from build123d import *

# Parameters (mm, degrees)
SKETCH1_W                    = 20
SKETCH1_H                    = 15
SKETCH1_W_2                  = 40
SKETCH1_H_2                  = 10
BOSS_EXTRUDE1_DEPTH          = 5
M3_CLEARANCE_HOLE1_OUTLINE_R = 1.7
M3_CLEARANCE_HOLE1_DEPTH     = 5
SKETCH4_W                    = 17
SKETCH4_H                    = 10
BOSS_EXTRUDE2_DEPTH          = 5
HOLE1_OUTLINE_R              = 2.2
HOLE1_DEPTH                  = 3
HOLE1_START                  = 3
HOLE1_2_OUTLINE_R            = 1.7
HOLE1_2_DEPTH                = 2
FILLET1_R                    = 4
FILLET2_R                    = 0.8


# Read off the part's stored shape, not the designer's step: M3 Clearance Hole1, Hole1
with BuildPart() as part:
    # Sketch1 → Boss-Extrude1 (new body)
    with BuildSketch(Plane.XY):
        with Locations((10, 17.5)):
            Rectangle(SKETCH1_W, SKETCH1_H)
        with Locations((20, 5)):
            Rectangle(SKETCH1_W_2, SKETCH1_H_2)
    extrude(amount=BOSS_EXTRUDE1_DEPTH)

    # M3 Clearance Hole1 outline → M3 Clearance Hole1 (cut)
    with BuildSketch(Plane.XY):
        with Locations((5, 17.5)):
            Circle(M3_CLEARANCE_HOLE1_OUTLINE_R)
        with Locations((15, 17.5)):
            Circle(M3_CLEARANCE_HOLE1_OUTLINE_R)
        with Locations((15, 5)):
            Circle(M3_CLEARANCE_HOLE1_OUTLINE_R)
        with Locations((35, 5)):
            Circle(M3_CLEARANCE_HOLE1_OUTLINE_R)
    extrude(amount=M3_CLEARANCE_HOLE1_DEPTH, mode=Mode.SUBTRACT)

    # Sketch4 → Boss-Extrude2 (add)
    with BuildSketch(Plane.XY.offset(5)):
        with Locations((-8.5, 5)):
            Rectangle(SKETCH4_W, SKETCH4_H)
    extrude(amount=-BOSS_EXTRUDE2_DEPTH)

    # Hole1 outline → Hole1 (cut)
    with BuildSketch(Plane.XY):
        with Locations((8, 5)):
            Circle(HOLE1_OUTLINE_R)
        with Locations((-12, 5)):
            Circle(HOLE1_OUTLINE_R)
    extrude(amount=HOLE1_DEPTH, mode=Mode.SUBTRACT)

    # Hole1 2 outline → Hole1 2 (cut)
    with BuildSketch(Plane.XY.offset(HOLE1_START)):
        with Locations((8, 5)):
            Circle(HOLE1_2_OUTLINE_R)
        with Locations((-12, 5)):
            Circle(HOLE1_2_OUTLINE_R)
    extrude(amount=HOLE1_2_DEPTH, mode=Mode.SUBTRACT)

    # Fillet1
    fillet1_edges = [part.edges().sort_by_distance(p)[0] for p in [
        (0, 25, 2.5),
        (20, 25, 2.5),
        (20, 10, 2.5),
        (40, 10, 2.5),
        (40, 0, 2.5),
        (0, 10, 2.5),
        (-17, 0, 2.5),
        (-17, 10, 2.5),
    ]]
    fillet(fillet1_edges, radius=FILLET1_R)

    # Fillet2
    fillet2_edges = [part.edges().sort_by_distance(p)[0] for p in [
        (21.171572875, 11.171572875, 0),
        (21.171572875, 11.171572875, 5),
        (-1.171572875, 11.171572875, 5),
        (-1.171572875, 11.171572875, 0),
        (-17, 5, 0),
        (-17, 5, 5),
        (0, 17.5, 5),
        (-8.5, 10, 5),
        (11.5, 0, 5),
        (40, 5, 5),
        (30, 10, 5),
        (20, 17.5, 5),
        (10, 25, 5),
        (1.171572875, 23.828427125, 5),
        (18.828427125, 23.828427125, 5),
        (38.828427125, 8.828427125, 5),
        (38.828427125, 1.171572875, 5),
        (-15.828427125, 8.828427125, 5),
        (-15.828427125, 1.171572875, 5),
        (11.5, 0, 0),
        (-8.5, 10, 0),
        (0, 17.5, 0),
        (10, 25, 0),
        (20, 17.5, 0),
        (30, 10, 0),
        (40, 5, 0),
        (1.171572875, 23.828427125, 0),
        (18.828427125, 23.828427125, 0),
        (38.828427125, 8.828427125, 0),
        (38.828427125, 1.171572875, 0),
        (-15.828427125, 8.828427125, 0),
        (-15.828427125, 1.171572875, 0),
    ]]
    fillet(fillet2_edges, radius=FILLET2_R)


solid = part.part
Part model, mm, in its own coordinate system. A direction names the side the tool comes from. Give positions to 0.01 mm unless a question says otherwise; leave off trailing zeros. Loops run counter-clockwise (first coordinate to the right, second up) from the corner with the lowest first, then second, coordinate; pieces in that order, holes last. Notation, with made-up numbers: M -23.5,30 L 18.5,30 A26 cw 18.5,59 Z; hole C 87.5,-4 d5. An arc over 180 degrees is marked long. Put each result on its own line as item: value. Start each with the question number.
1) Probe probe 1 along Y at (x, z) = (14.5, 4.65); probe 2 along Y at (x, z) = (15, 3.35); probe 3 along X at (y, z) = (4.25, 1.35). List the from-to ranges inside material, lowest first.
2) Pull direction X, two halves, no side cores. Call faces 1 (the flat face through (6, 5, 3)), 2 (the flat face through (11, 0, 3)), 3 (the flat face through (-17, 5, 3)): +X half, -X half, draft (parallel to the pull), parting line (faces both ways), or undercut.
3) Saw through at A-A (x = 5). List the corners of the cut face in (y, z).
4) Saw through at C-C (x = 15). List the corners of the cut face in (y, z).
5) Saw through at D-D (y = 17.5). List the corners of the cut face in (x, z), then the cut area to 3 significant figures.
6) 3-axis set-ups, long thin cutter, end or side, ignore diameter. For faces 4 (the cylindrical face through (-9.968, 4.157, 1.479)), 5 (the flat face through (11, 10, 0)): which of +Z, -Z, +X, -X, +Y, -Y reach the whole face in a straight line?
7) Flat gauge pins, fed straight in: pin 1 (2.5 mm diameter, centred on x = 8, y = 5, fed in from +Z); pin 2 (1 mm diameter, centred on y = 16.5, z = 3, fed in from -X); pin 3 (4 mm diameter, centred on x = 15, y = 5, fed in from +Z); pin 4 (2.5 mm diameter, centred on x = 28.5, z = 2, fed in from +Y). Where does each tip first touch, or does it go through?
8) Saw through at B-B (y = 5). State how many separate pieces and enclosed holes the cut face has, then the cut area to 3 significant figures.
Numbers:
1. probe 1: 0.14 to 3.38, 6.62 to 15.88, 19.12 to 24.86
1. probe 2: 0 to 3.3, 6.7 to 15.8, 19.2 to 25
1. probe 3: -17 to -14.07, -9.93 to 5.93, 10.07 to 13.47, 16.53 to 33.47, 36.53 to 40
2. face 1: undercut
2. face 2: draft
2. face 3: -X half
3. outline: M 0,0.8 A0.8 ccw 0.8,0 L 15.8,0 L 15.8,5 L 0.8,5 A0.8 ccw 0,4.2 Z; M 19.2,0 L 24.2,0 A0.8 ccw 25,0.8 L 25,4.2 A0.8 ccw 24.2,5 L 19.2,5 Z
4. outline: M 0,0.8 A0.8 ccw 0.8,0 L 3.3,0 L 3.3,5 L 0.8,5 A0.8 ccw 0,4.2 Z; M 6.7,0 L 15.8,0 L 15.8,5 L 6.7,5 Z; M 19.2,0 L 24.2,0 A0.8 ccw 25,0.8 L 25,4.2 A0.8 ccw 24.2,5 L 19.2,5 Z
5. outline: M 0,0.8 A0.8 ccw 0.8,0 L 3.3,0 L 3.3,5 L 0.8,5 A0.8 ccw 0,4.2 Z; M 6.7,0 L 13.3,0 L 13.3,5 L 6.7,5 Z; M 16.7,0 L 19.2,0 A0.8 ccw 20,0.8 L 20,4.2 A0.8 ccw 19.2,5 L 16.7,5 Z
5. area: 65.5 mm^2
6. face 4: -Z
6. face 5: -Z, +X, -X, +Y, -Y
7. pin 1: through
7. pin 2: x = 0
7. pin 3: z = 5
7. pin 4: y = 10
8. separate pieces: 5
8. enclosed holes: 0
8. area: 210 mm^2
